Build history of the part. All positions in model axes, mm. Face numbers are marked on the shaded views. A direction names the side the tool comes from. Round coordinates to 2 decimals unless told otherwise and drop trailing zeros. Order: outer loops, then holes, each group sorted by start corner. A loop starts at its lowest first (then second) coordinate and runs counter-clockwise, first axis right, second up. Notation, with made-up numbers: (42.5, -17) -> (90.5, -17) arc R11 cw to (90.5, -8) -> close; hole circle Ø5 at (-35.75, 29.5). An arc over 180 degrees is marked (long way). Answer as a JSON object with one key per item and string values.
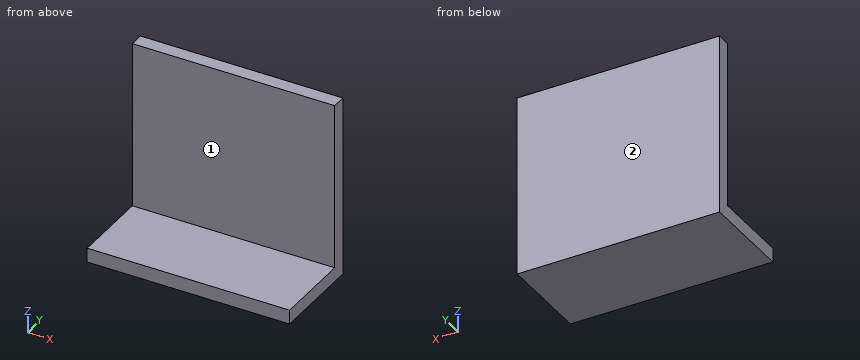
from build123d import *

# Parameters (mm, degrees)
F0_W     = 565.15
F0_H     = 101.6
F1_DEPTH = 1447.8
F2_W     = 101.6
F2_H     = 1295.4
F3_DEPTH = 1447.8


with BuildPart() as f1:
    # F0 (on Right) → F1 (new body)
    with BuildSketch(Plane.YZ):
        with Locations((71.596854, -22.620682)):
            Rectangle(F0_W, F0_H)
    extrude(amount=F1_DEPTH)

    # F2 (on Right) → F3 (join)
    with BuildSketch(Plane.YZ):
        with Locations((404.971854, 574.279318)):
            Rectangle(F2_W, F2_H)
    extrude(amount=F3_DEPTH)


solid = f1.part
1) Probe L1, parallel to Y at x = 301, z = 326.5; L2, parallel to Z at x = 1305, y = -160. List the from-to ranges inside material, lowest first. Write a range as from..to.
Checked values:
{"L1": "y = 354.17..455.77", "L2": "z = -73.42..28.18"}
2) Which spindle directions (+Z, -Z, +X, -X, +Y, -Y) get a long thin tool onto all of the face, cutting with end or side? Do the marked faces 1 and 2. Say none if no direction does.
Checked values:
{"face 1": "+Z, +X, -X, -Y", "face 2": "+Z, -Z, +X, -X, +Y"}
3) Flat gauge pins, fed straight in: pin 1 Ø10 at (x, y) = (1053, 135.5) entering from +Z; pin 2 Ø8 at (x, z) = (358, 756.5) entering from -Y. Where does each tip first touch, or does it go through?
Checked values:
{"pin 1": "stops at z = 28.18", "pin 2": "stops at y = 354.17"}
4) Cut at A-A, the plane x = 497. Give the cut face in (y, z), plus the area to 3 significant figures.
Checked values:
{"outline": "(-210.98, -73.42) -> (455.77, -73.42) -> (455.77, 1221.98) -> (354.17, 1221.98) -> (354.17, 28.18) -> (-210.98, 28.18) -> close", "area": "189,000 mm²"}
5) Cut at B-B, the plane z = 332. Give the cut face in (x, y), plus the area to 3 significant figures.
Checked values:
{"outline": "(0, 354.17) -> (1447.8, 354.17) -> (1447.8, 455.77) -> (0, 455.77) -> close", "area": "147,000 mm²"}
6) Cut at C-C, the plane y = 290. Give the cut face in (x, z), plus the area to 3 significant figures.
Checked values:
{"outline": "(0, -73.42) -> (1447.8, -73.42) -> (1447.8, 28.18) -> (0, 28.18) -> close", "area": "147,000 mm²"}
